```python
from build123d import *

# Parameters (mm, degrees)
F0_R     = 42.5
F0_R_2   = 3.5
F1_DEPTH = 20
F2_START = 18
F2_DEPTH = 2
F3_SIZE  = 1.414
F4_SIZE  = 1.414


with BuildPart() as f1:
    # F0 (on Top) → F1 (new body)
    with BuildSketch(Plane.XY):
        Circle(F0_R)
        Polygon((-4.9074772881, -13.5), (4.9074772881, -13.5), (9.8149545762, -22), (4.9074772881, -30.5), (-4.9074772881, -30.5), (-9.8149545762, -22), align=None, mode=Mode.SUBTRACT)
        Polygon((-14.1450815951, -2.5), (-9.237604307, -11), (-14.1450815951, -19.5), (-23.9600361714, -19.5), (-28.8675134595, -11), (-23.9600361714, -2.5), align=None, mode=Mode.SUBTRACT)
        Polygon((9.237604307, -11), (14.1450815951, -2.5), (23.9600361714, -2.5), (28.8675134595, -11), (23.9600361714, -19.5), (14.1450815951, -19.5), align=None, mode=Mode.SUBTRACT)
        Polygon((-9.237604307, 11), (-14.1450815951, 2.5), (-23.9600361714, 2.5), (-28.8675134595, 11), (-23.9600361714, 19.5), (-14.1450815951, 19.5), align=None, mode=Mode.SUBTRACT)
        Circle(F0_R_2, mode=Mode.SUBTRACT)
        Polygon((14.1450815951, 2.5), (9.237604307, 11), (14.1450815951, 19.5), (23.9600361714, 19.5), (28.8675134595, 11), (23.9600361714, 2.5), align=None, mode=Mode.SUBTRACT)
        Polygon((9.8149545762, 22), (4.9074772881, 13.5), (-4.9074772881, 13.5), (-9.8149545762, 22), (-4.9074772881, 30.5), (4.9074772881, 30.5), align=None, mode=Mode.SUBTRACT)
    extrude(amount=F1_DEPTH)

    # F0 (on Top) → F2 (join)
    with BuildSketch(Plane.XY.offset(F2_START)):
        Polygon((-23.9600361714, 2.5), (-14.1450815951, 2.5), (-9.237604307, 11), (-14.1450815951, 19.5), (-23.9600361714, 19.5), (-28.8675134595, 11), align=None)
        Polygon((-4.9074772881, 13.5), (4.9074772881, 13.5), (9.8149545762, 22), (4.9074772881, 30.5), (-4.9074772881, 30.5), (-9.8149545762, 22), align=None)
        Polygon((14.1450815951, 19.5), (9.237604307, 11), (14.1450815951, 2.5), (23.9600361714, 2.5), (28.8675134595, 11), (23.9600361714, 19.5), align=None)
        Polygon((23.9600361714, -2.5), (14.1450815951, -2.5), (9.237604307, -11), (14.1450815951, -19.5), (23.9600361714, -19.5), (28.8675134595, -11), align=None)
        Polygon((9.8149545762, -22), (4.9074772881, -13.5), (-4.9074772881, -13.5), (-9.8149545762, -22), (-4.9074772881, -30.5), (4.9074772881, -30.5), align=None)
        Polygon((-14.1450815951, -19.5), (-9.237604307, -11), (-14.1450815951, -2.5), (-23.9600361714, -2.5), (-28.8675134595, -11), (-23.9600361714, -19.5), align=None)
    extrude(amount=F2_DEPTH)

    # F3
    f3_edges = [f1.edges().sort_by_distance(p)[0] for p in [
        (-42.5, 0, 20),
    ]]
    chamfer(f3_edges, length=F3_SIZE)

    # F4
    f4_edges = [f1.edges().sort_by_distance(p)[0] for p in [
        (-42.5, 0, 0),
    ]]
    chamfer(f4_edges, length=F4_SIZE)


solid = f1.part
```
For this review, take the finished solid that the model builds, in its own axes (mm). A direction names the side the tool comes from. Give positions to 0.01 mm unless a question says otherwise; leave off trailing zeros. Write each loop counter-clockwise with the first axis right and the second up, starting at its lowest first coordinate (ties: lowest second). Pieces come first, ordered by that corner, then holes. Notation, with made-up numbers: M 48,74 L 90,74 A19 cw 90,106 Z; hole C -37.5,37.25 d6. An arc over 180 degrees is marked long. Answer as CSV lines item,"result".
1. Consider section C-C, the plane z = 5.5. Count the separate pieces of the cut face and the enclosed holes in it, then the cut area to 3 significant figures.
Findings:
separate pieces,"1"
enclosed holes,"7"
area,"4,130 mm2"
2. For faces 3 (the flat face through (-11.657, 6.809, 8.874)), 4 (the flat face through (-1, -9, 0)), list the 3-axis set-ups (+Z, -Z, +X, -X, +Y, -Y) from which the entire face can be reached by the end or side of a thin tool; tool diameter is ignored.
Findings:
face 3,"-Z"
face 4,"-Z, +X, -X, +Y, -Y"
3. For pin 1 (3 mm diameter, centred on x = 21, z = 8.5, fed in from -Y); pin 2 (11 mm diameter, centred on x = 2.5, z = 5, fed in from -Y); pin 3 (5 mm diameter, centred on x = -1.5, z = 11.5, fed in from +Y), all flat-tipped, find the tip position at first contact; note any pin that passes through.
Findings:
pin 1,"stops at y = -37.76"
pin 2,"stops at y = -42.5"
pin 3,"stops at y = 42.5"
4. Draft analysis for pull direction Y (two halves, no side actions). For faces 1 (the flat face through (-1, -9, 20)), 2 (the flat face through (0, 30.5, 9)), state which applies: +Y half, -Y half, draft (parallel to the pull), parting line (faces both ways), or undercut.
Findings:
face 1,"draft"
face 2,"undercut"
5. Consider section B-B, the plane x = 0. Write out the cut boundary in (y, z), then the cut area to 3 significant figures.
Findings:
outline,"M -42.5,1.41 L -41.09,0 L -30.5,0 L -30.5,18 L -13.5,18 L -13.5,0 L -3.5,0 L -3.5,20 L -41.09,20 L -42.5,18.59 Z; M 3.5,0 L 13.5,0 L 13.5,18 L 30.5,18 L 30.5,0 L 41.09,0 L 42.5,1.41 L 42.5,18.59 L 41.09,20 L 3.5,20 Z"
area,"944 mm2"
6. Consider section A-A, the plane y = 0. Write out the cut boundary in (x, z), then the cut area to 3 significant figures.
Findings:
outline,"M -42.5,1.41 L -41.09,0 L -3.5,0 L -3.5,20 L -41.09,20 L -42.5,18.59 Z; M 3.5,0 L 41.09,0 L 42.5,1.41 L 42.5,18.59 L 41.09,20 L 3.5,20 Z"
area,"1,560 mm2"
7. Wall thickness on line 1 (Y direction, x = 0, z = 11.25); line 2 (X direction, y = 15.5, z = 5.25); line 3 (X direction, y = 17, z = 5.25): over which ranges is each line inside the solid? List them lowest first.
Findings:
line 1,"y = -42.5 to -30.5, -13.5 to -3.5, 3.5 to 13.5, 30.5 to 42.5"
line 2,"x = -39.57 to -26.27, -11.84 to -6.06, 6.06 to 11.84, 26.27 to 39.57"
line 3,"x = -38.95 to -25.4, -12.7 to -6.93, 6.93 to 12.7, 25.4 to 38.95"
